Source: three-view drawing plus pictorial views. Frame: mm from the lowest corner of the part. Give positions to 0.01 mm unless a question says otherwise; leave off trailing zeros. Order: outer loops, then holes, each group sorted by start corner. A loop starts at its lowest first (then second) coordinate and runs counter-clockwise, first axis right, second up. Notation, with made-up numbers: (-8, -35.5) -> (0, -35.5) arc R10 cw to (0, -19.5) -> close; hole circle Ø2 at (26.25, -24.75). An arc over 180 degrees is marked (long way). Write item = value, one per line.
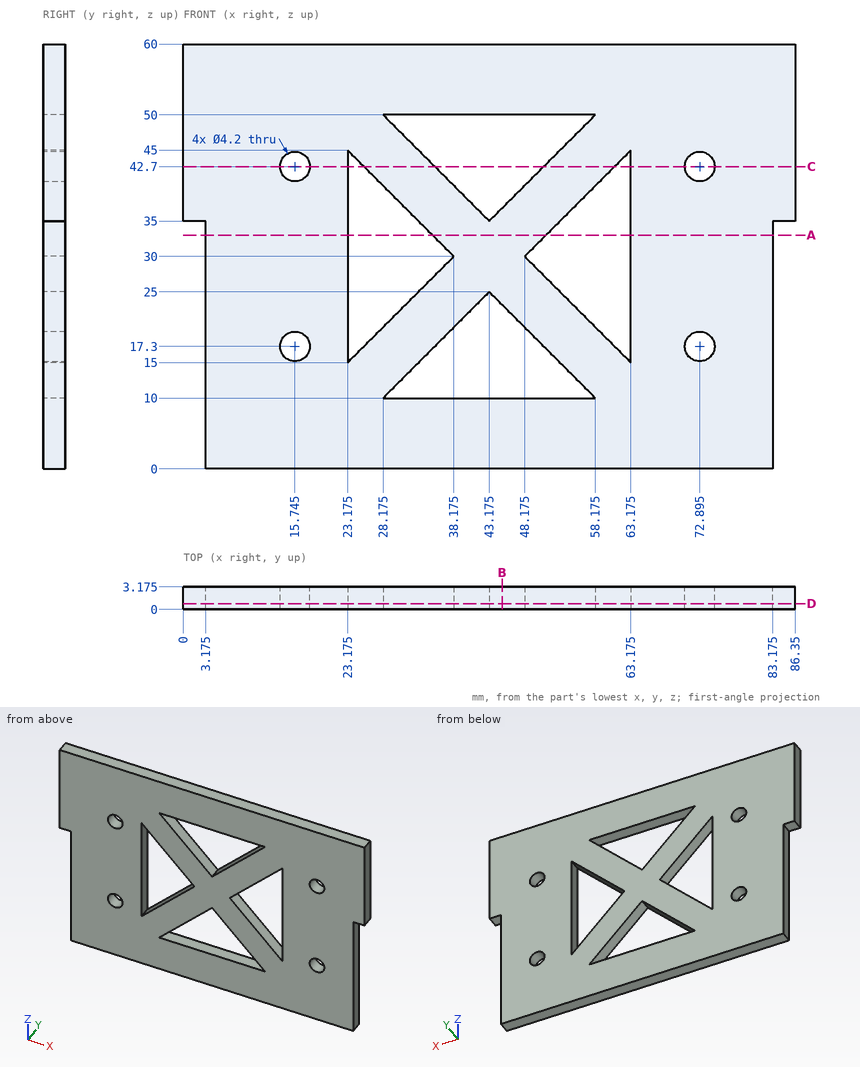
1) Line query: line 1 (Z direction, x = 16, y = 0.65); line 2 (X direction, y = 2, z = 42.7) (3 decimals); line 3 (Z direction, x = 29, y = 0.2) (3 decimals). Output: solid intervals per line, ascending. Write a range as from..to.
Check sheet entries:
line_1 = 0..15.22, 19.38..40.62, 44.78..60
line_2 = 0..13.645, 17.845..23.175, 25.475..35.475, 50.875..60.875, 63.175..70.795, 74.995..86.35
line_3 = 0..10, 10.825..20.825, 39.175..49.175, 50..60
2) Section query D-D (y = 0.8). Count the separate pieces of the cut face and the enclosed holes in it, plus the area to 3 significant figures.
Check sheet entries:
separate_pieces = 1
enclosed_holes = 8
area = 4,000 mm²
3) Section query A-A (z = 33). Output: boundary loops of the cut face in (x, y) (3 decimals), plus the area to 3 significant figures.
Check sheet entries:
outline = (3.175, 0) -> (23.175, 0) -> (23.175, 3.175) -> (3.175, 3.175) -> close; (35.175, 0) -> (51.175, 0) -> (51.175, 3.175) -> (35.175, 3.175) -> close; (63.175, 0) -> (83.175, 0) -> (83.175, 3.175) -> (63.175, 3.175) -> close
area = 178 mm²
4) First-contact query: P1, Ø6.5, axis at x = 72.895, z = 42.7, coming from the +Y side (3 decimals); P2, Ø1, axis at y = 1.5, z = 29.5, coming from the -X side (3 decimals); P3, Ø1, axis at y = 2, z = 10, coming from the +X side (3 decimals); P4, Ø1, axis at x = 2.5, y = 1, coming from the -Z side. Flat tips, straight axial feed; report the tip coordinate or a pass-through.
Check sheet entries:
P1 = 3.175
P2 = 3.175
P3 = 83.175
P4 = 35
5) Section query C-C (z = 42.7). Output: boundary loops of the cut face in (x, y) (3 decimals).
Check sheet entries:
outline = (0, 0) -> (13.645, 0) -> (13.645, 3.175) -> (0, 3.175) -> close; (17.845, 0) -> (23.175, 0) -> (23.175, 3.175) -> (17.845, 3.175) -> close; (25.475, 0) -> (35.475, 0) -> (35.475, 3.175) -> (25.475, 3.175) -> close; (50.875, 0) -> (60.875, 0) -> (60.875, 3.175) -> (50.875, 3.175) -> close; (63.175, 0) -> (70.795, 0) -> (70.795, 3.175) -> (63.175, 3.175) -> close; (74.995, 0) -> (86.35, 0) -> (86.35, 3.175) -> (74.995, 3.175) -> close
6) Section query B-B (x = 45). Output: boundary loops of the cut face in (y, z) (3 decimals), plus the area to 3 significant figures.
Check sheet entries:
outline = (0, 0) -> (3.175, 0) -> (3.175, 10) -> (0, 10) -> close; (0, 23.175) -> (3.175, 23.175) -> (3.175, 36.825) -> (0, 36.825) -> close; (0, 50) -> (3.175, 50) -> (3.175, 60) -> (0, 60) -> close
area = 107 mm²
